Verification items for the finished model (mm, model axes). Round coordinates to 2 decimals unless told otherwise and drop trailing zeros. Write each loop counter-clockwise with the first axis right and the second up, starting at its lowest first coordinate (ties: lowest second). Pieces come first, ordered by that corner, then holes. Notation, with made-up numbers: M 37,-0.5 L 60,-0.5 A30 ccw 60,21.5 Z; hole C -32,-12.5 d3. An arc over 180 degrees is marked long. One line per question, with ' | ' between items. Start each with the question number.
Q1. Release check for a two-part mould opening along X. For faces 1 (the face through (-12.83, -0.32, -0.6)), 2 (the face through (0.7, -0.3, -45.5)), 3 (the face through (0, -0.63, -25)), 4 (the face through (0.5, -0.3, -4.5)) record: released by +X, released by -X, zero draft, split by the parting line, or undercut.
Q2. Cross-section at A-A (y = -0.45). Record the boundary of the cut face in (x, z).
Q3. Thickness scan on line 1 along Z through (x, y) = (13.75, -0.35); line 2 along Z through (x, y) = (-1, -0.45). Record the ranges inside material, lowest first. Write a range as from..to.
Q4. Cross-section at B-B (x = 1.5). Record the boundary of the cut face in (y, z).
from build123d import *

# Parameters (mm, degrees)
EXTRUDE_1_DEPTH = 0.63
FILLET_3_R      = 2


with BuildPart() as part:
    # Sketch 1 → Extrude 1 (new body)
    with BuildSketch(Plane(origin=(0, 0, 0), x_dir=(1, 0, 0), z_dir=(0, 1, 0))):
        with BuildLine():
            Line((5.101078805, 0), (14.601078805, 0))
            Line((14.601078805, 0), (14.601078805, 50))
            Line((14.601078805, 50), (5.101078805, 50))
            ThreePointArc((5.101078805, 50), (0.601078805, 45.5), (-3.898921195, 50))
            Line((-3.898921195, 50), (-13.398921195, 50))
            Line((-13.398921195, 50), (-13.398921195, 0))
            Line((-13.398921195, 0), (-3.898921195, 0))
            ThreePointArc((-3.898921195, 0), (0.601078805, 4.5), (5.101078805, 0))
        make_face()
    extrude(amount=-EXTRUDE_1_DEPTH)

    # Fillet 3
    fillet_3_edges = [part.edges().sort_by_distance(p)[0] for p in [
        (-13.398921195, -0.315, 0),
        (-13.398921195, -0.315, -50),
        (14.601078805, -0.315, -50),
        (14.601078805, -0.315, 0),
    ]]
    fillet(fillet_3_edges, radius=FILLET_3_R)


solid = part.part
Determined:
1) face 1: released by -X | face 2: undercut | face 3: zero draft | face 4: undercut
2) outline: M -13.4,-48 A2 ccw -11.4,-50 L -3.9,-50 A4.5 cw 5.1,-50 L 12.6,-50 A2 ccw 14.6,-48 L 14.6,-2 A2 ccw 12.6,0 L 5.1,0 A4.5 cw -3.9,0 L -11.4,0 A2 ccw -13.4,-2 Z
3) line 1: z = -49.64..-0.36 | line 2: z = -45.79..-4.21
4) outline: M -0.63,-45.59 L 0,-45.59 L 0,-4.41 L -0.63,-4.41 Z
